Read the model definition and answer for the solid it produces. Units are mm, in the model's axes. Face numbers are marked on the shaded views. A direction names the side the tool comes from. Coordinates: 2 decimals unless noted, no trailing zeros. Loops run counter-clockwise (first coordinate to the right, second up) from the corner with the lowest first, then second, coordinate; pieces in that order, holes last. Notation, with made-up numbers: (40, -5) - (48, -5) arc R30 cw to (48, 21) - close; hole circle Ø3 at (82.5, 59.5). An arc over 180 degrees is marked (long way). Use one line per item in the form item = value. Start each with the question number.
1) A cutting plane is placed at D-D (z = 39). Give the vertices of the cut face in (x, y).
2) The mould has two halves that part along Y. Classify the marked faces 4, 5 and 6: released by +Y, released by -Y, zero draft, split by the parting line, or undercut.
3) Which of the six approach directions +Z, -Z, +X, -X, +Y, -Y give full straight-line access (tool end or side, diameter ignored) to the marked faces 1, 2 and 3?
4) A cutting plane is placed at C-C (x = -16.25). State how many separate pieces and enclosed holes the cut face has, and give its area (3 significant figures).
5) Each of these flat-tipped pins is pushed along its axis until it touches: P1, Ø5, axis at y = 8, z = 86, coming from the -X side; P2, Ø3, axis at y = 15, z = 2, coming from the -X side. Where does it stop, or does it pass through?
6) A cutting plane is placed at B-B (y = 4). Give the vertices of the cut face in (x, z), and give its area (3 significant figures).
7) A cutting plane is placed at A-A (y = 29.5). Give the vertices of the cut face in (x, z).
8) Consider line 1 (Z direction, x = -6.75, y = 42); line 2 (Y direction, x = -4, z = 86); line 3 (Z direction, x = -3.5, y = 28.5). Determine where each line is inside the solid, lowest interval first.
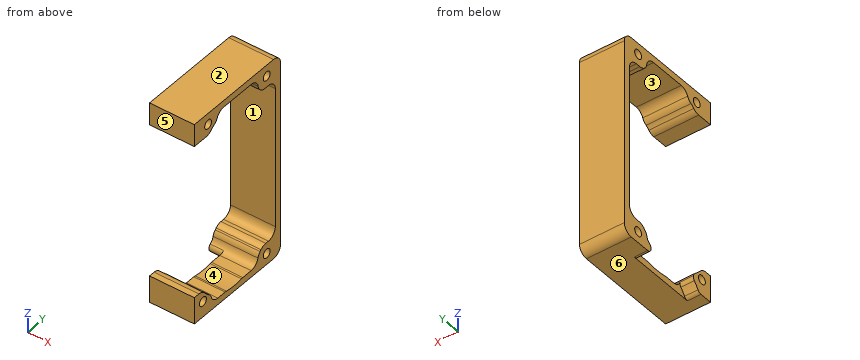
Autodesk Inventor part; units mm, degrees
ref_plane "YZ Plane" through (0, 0, 0) normal (1, 0, 0) x (0, 1, 0)
ref_plane "XZ Plane" through (0, 0, 0) normal (0, 1, 0) x (-1, 0, 0)
ref_plane "XY Plane" through (0, 0, 0) normal (0, 0, 1) x (1, 0, 0)
sketch "Sketch2" plane through (0, 0, 0) normal (1, 0, 0) x (0, 1, 0)
  line L0 (0, 0) -> (50, 0)
  line L1 (50, 0) -> (50, 91)
  line L2 (50, 91) -> (0, 91)
  line L3 (0, 91) -> (0, 0)
  dimension "d39" = 50
  dimension "d40" = 91
extrude "Extrusion2" add sketch "Sketch2" against normal blind 20
sketch "Sketch3" plane through (-20, 0, 0) normal (-1, 0, 0) x (0, 0, 1)
  line L0 (0, 0) -> (91, 0)
  line L1 (0, 50) -> (0, 0)
  point P0 (7, 5)
  point P1 (5, 42)
  point P2 (86, 42)
  point P3 (86, 8)
  dimension "d43" = 8
  dimension "d44" = 86
  dimension "d45" = 42
  dimension "d46" = 5
  dimension "d47" = 7
  dimension "d48" = 5
hole "Hole1" at (-20, 5, 7) at (-20, 42, 5) at (-20, 42, 86) at (-20, 8, 86) direction (1, 0, 0) diameter 4 end through all
fillet "Fillet8" radius 4 2 edges at (-10, 50, 0) (-10, 50, 91)
sketch "Sketch4" plane through (-20, 0, 0) normal (-1, 0, 0) x (0, 0, 1)
  line L0 (91, 0) -> (0, 0)
  line L1 (12, 0) -> (81, 0)
  line L2 (81, 13) -> (81, 0)
  line L3 (81, 13) -> (88, 13)
  line L4 (88, 13) -> (88, 37)
  line L5 (88, 37) -> (81, 37)
  line L6 (81, 37) -> (81, 47)
  line L7 (81, 47) -> (10, 47)
  line L8 (10, 47) -> (10, 37)
  line L9 (10, 37) -> (3, 37)
  line L10 (3, 37) -> (3, 10)
  line L11 (0, 46) -> (0, 0)
  line L12 (3, 10) -> (12, 10)
  line L13 (12, 10) -> (12, 0)
  line L14 (0, 0) -> (91, 0)
  dimension "d57" = 3
  dimension "d58" = 88
  dimension "d59" = 47
  dimension "d60" = 10
  dimension "d61" = 37
  dimension "d62" = 81
  dimension "d63" = 13
  dimension "d67" = 12
  dimension "d68" = 10
extrude "Extrusion3" cut sketch "Sketch4" against normal through all
sketch "Sketch5" plane through (-20, 0, 0) normal (-1, 0, 0) x (0, 0, 1)
  circle A0 centre (25, 23) radius 22.5
  circle A1 centre (78, 14) radius 6
  point P0 (0, 0)
  dimension "d69" = 25
  dimension "d70" = 23
  dimension "d71" = 45
  dimension "d75" = 12
  dimension "d76" = 78
  dimension "d77" = 14
extrude "Extrusion4" cut sketch "Sketch5" against normal through all
fillet "Fillet9" radius 4 15 edges at (-10, 37, 3) (-10, 18.283, 3) (-10, 27.717, 3) (-10, 10, 3) (-10, 10, 6.6356) (-10, 4.6356, 12) (-10, 37, 7.3861) (-10, 39.7705, 10) (-10, 47, 10) (-10, 47, 81) (-10, 37, 81) (-10, 37, 88) (-10, 13, 88) (-10, 13, 83.9161) (-10, 8.8038, 81)
sketch "Sketch6" plane through (-20, 0, 0) normal (-1, 0, 0) x (0, 0, 1)
  circle A0 centre (-7.25, 21) radius 16
  point P0 (0, 0)
  dimension "d78" = 32
  dimension "d79" = 21
  dimension "d80" = 7.25
extrude "Extrusion5" cut sketch "Sketch6" against normal blind 6
fillet "Fillet10" radius 2 4 edges at (-17, 35.2632, 0) (-17, 6.7368, 0) (-17, 33.2776, 3.0096) (-17, 10.3732, 4.7112)
properties part number "One Motor Gearbox Cover"
Found:
q1.outline = (-20, 47) - (0, 47) - (0, 50) - (-20, 50) - close
q2.face_4 = undercut
q2.face_5 = released by -Y
q2.face_6 = zero draft
q3.face_1 = +X, -X, -Y
q3.face_2 = +Z, +X, -X, +Y, -Y
q3.face_3 = +X, -X
q4.separate_pieces = 2
q4.enclosed_holes = 4
q4.area = 719 mm^2
q5.P1 = -20
q5.P2 = -14
q6.outline = (-20, 0) - (0, 0) - (0, 5.27) - (-20, 5.27) - close; (-20, 8.73) - (0, 8.73) - (0, 11.77) - (-20, 11.77) - close; (-20, 81) - (0, 81) - (0, 91) - (-20, 91) - close
q6.area = 366 mm^2
q7.outline = (-20, 88) - (0, 88) - (0, 91) - (-20, 91) - close; (-14, 0) - (0, 0) - (0, 3) - (-14, 3) - close
q8.line_1 = 0 to 3, 7 to 10, 81 to 84, 88 to 91
q8.line_2 = 0 to 6, 10 to 13.54, 36.53 to 40, 44 to 50
q8.line_3 = 0 to 3, 88 to 91
